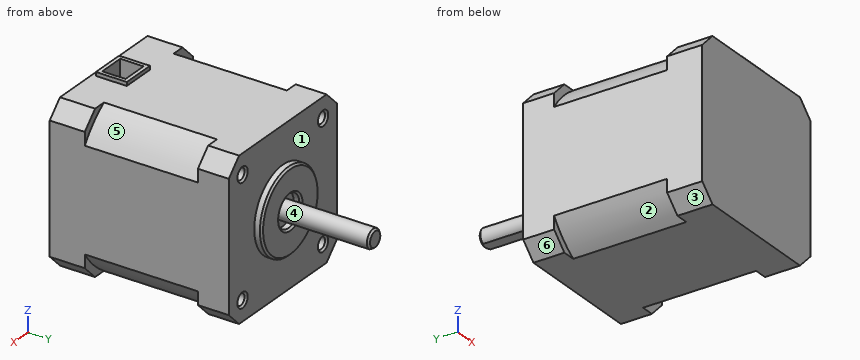
from build123d import *

# Parameters (mm, degrees)
SKETCH1_W           = 42
SKETCH1_H           = 42
BOSS_EXTRUDE1_DEPTH = 47.5
CHAMFER1_SIZE       = 4
SKETCH2_R           = 11.1
SKETCH2_R_2         = 4.25
BOSS_EXTRUDE2_DEPTH = 2
SKETCH4_R           = 2.5
BOSS_EXTRUDE3_DEPTH = 24.5
CHAMFER2_SIZE       = 0.5
CUT_EXTRUDE1_DEPTH  = 18
SKETCH6_R           = 1.5
CUT_EXTRUDE2_DEPTH  = 5
CUT_EXTRUDE3_START  = 9.3
SKETCH7_R           = 36.852304789
SKETCH7_R_2         = 25
CUT_EXTRUDE3_DEPTH  = 30
SKETCH8_W           = 9
SKETCH8_H           = 8.197254607
SKETCH8_W_2         = 7
SKETCH8_H_2         = 6.197254607
EXTRUDE_THIN1_DEPTH = 1
SKETCH9_W           = 7
SKETCH9_H           = 6.197254607
CUT_EXTRUDE4_DEPTH  = 5
CHAMFER3_SIZE       = 0.5


with BuildPart() as part:
    # Sketch1 → Boss-Extrude1 (new body)
    with BuildSketch(Plane(origin=(0, 0, 0), x_dir=(1, 0, 0), z_dir=(0, 1, 0))):
        Rectangle(SKETCH1_W, SKETCH1_H)
    extrude(amount=BOSS_EXTRUDE1_DEPTH)

    # Chamfer1
    chamfer1_edges = [part.edges().sort_by_distance(p)[0] for p in [
        (21, 23.75, 21),
        (-21, 23.75, 21),
        (-21, 23.75, -21),
        (21, 23.75, -21),
    ]]
    chamfer(chamfer1_edges, length=CHAMFER1_SIZE)

    # Sketch2 → Boss-Extrude2 (add)
    with BuildSketch(Plane.XZ.offset(-47.5)):
        with Locations(Location((0, 0, 0), (0, 0, 270))):
            Circle(SKETCH2_R)
        with Locations(Location((0, 0, 0), (0, 0, 270))):
            Circle(SKETCH2_R_2, mode=Mode.SUBTRACT)
    extrude(amount=-BOSS_EXTRUDE2_DEPTH)

    # Sketch4 → Boss-Extrude3 (add)
    with BuildSketch(Plane(origin=(0, 47.5, 0), x_dir=(1, 0, 0), z_dir=(0, 1, 0))):
        with Locations(Location((0, 0, 0), (0, 0, 270))):
            Circle(SKETCH4_R)
    extrude(amount=BOSS_EXTRUDE3_DEPTH)

    # Chamfer2
    chamfer2_edges = [part.edges().sort_by_distance(p)[0] for p in [
        (0, 72, -2.5),
    ]]
    chamfer(chamfer2_edges, length=CHAMFER2_SIZE)

    # Sketch5 → Cut-Extrude1 (cut)
    with BuildSketch(Plane(origin=(0, 72, 0), x_dir=(1, 0, 0), z_dir=(0, 1, 0))):
        Polygon((-1.867188484, 2), (1.973628394, 2), (0.053219955, 2.996371605), align=None)
    extrude(amount=-CUT_EXTRUDE1_DEPTH, mode=Mode.SUBTRACT)

    # Sketch6 → Cut-Extrude2 (cut)
    with BuildSketch(Plane(origin=(0, 47.5, 0), x_dir=(1, 0, 0), z_dir=(0, 1, 0))):
        with Locations(Location((-15.637811111, 15.662146765, 0), (0, 0, 270))):
            Circle(SKETCH6_R)
        with Locations(Location((15.662146765, 15.637811111, 0), (0, 0, 270))):
            Circle(SKETCH6_R)
        with Locations(Location((15.637811111, -15.662146765, 0), (0, 0, 270))):
            Circle(SKETCH6_R)
        with Locations(Location((-15.662146765, -15.637811111, 0), (0, 0, 270))):
            Circle(SKETCH6_R)
    extrude(amount=-CUT_EXTRUDE2_DEPTH, mode=Mode.SUBTRACT)

    # Sketch7 → Cut-Extrude3 (cut)
    with BuildSketch(Plane(origin=(0, 0, 0), x_dir=(1, 0, 0), z_dir=(0, 1, 0)).offset(CUT_EXTRUDE3_START)):
        Circle(SKETCH7_R)
        Circle(SKETCH7_R_2, mode=Mode.SUBTRACT)
    extrude(amount=CUT_EXTRUDE3_DEPTH, mode=Mode.SUBTRACT)

    # Sketch8 → Extrude-Thin1 (add)
    with BuildSketch(Plane.XY.offset(21)):
        with Locations((0, 5.081594665)):
            Rectangle(SKETCH8_W, SKETCH8_H)
        with Locations((0, 5.081594665)):
            Rectangle(SKETCH8_W_2, SKETCH8_H_2, mode=Mode.SUBTRACT)
    extrude(amount=EXTRUDE_THIN1_DEPTH)

    # Sketch9 → Cut-Extrude4 (cut)
    with BuildSketch(Plane.XY.offset(21)):
        with Locations((0, 5.081594665)):
            Rectangle(SKETCH9_W, SKETCH9_H)
    extrude(amount=-CUT_EXTRUDE4_DEPTH, mode=Mode.SUBTRACT)

    # Chamfer3
    chamfer3_edges = [part.edges().sort_by_distance(p)[0] for p in [
        (0, 49.5, 11.1),
        (0, 49.5, 4.25),
        (-15.637811111, 47.5, -17.162146765),
        (15.662146765, 47.5, -17.137811111),
        (15.637811111, 47.5, 14.162146765),
        (-15.662146765, 47.5, 14.137811111),
    ]]
    chamfer(chamfer3_edges, length=CHAMFER3_SIZE)


solid = part.part
Source: CAD feature listing. Evaluate the final solid. Frame: model axes, mm. Face numbers are marked on the shaded views. A direction names the side the tool comes from. Round coordinates to 2 decimals unless told otherwise and drop trailing zeros. Loops run counter-clockwise (first coordinate to the right, second up) from the corner with the lowest first, then second, coordinate; pieces in that order, holes last. Notation, with made-up numbers: (1.5, 28) - (40.5, 28) arc R21 cw to (40.5, 54) - close; hole circle Ø7 at (71, 22.5). An arc over 180 degrees is marked (long way). Write item = value, one per line. Start each with the question number.
(1) Pull-direction query (Y, two-part tool) for the marked faces 1, 2 and 3; classes: +Y half, -Y half, draft (parallel to the pull), parting line (faces both ways), or undercut.
(2) Pin query (flat end, axial travel): pin 1 (12 mm diameter, centred on x = 12, z = -9.5, fed in from +Y); pin 2 (12 mm diameter, centred on y = 57.5, z = -13, fed in from -X); pin 3 (1.1 mm diameter, centred on y = 6.5, z = 21.5, fed in from -X); pin 4 (1.5 mm diameter, centred on x = -15.5, z = 16, fed in from +Y). Return the tip coordinate at first contact, or that it passes through.
(3) Section query A-A, the plane y = 26.5. Output: boundary loops of the cut face in (x, z), plus the area to 3 significant figures.
(4) Section query B-B, the plane z = 0. Output: boundary loops of the cut face in (x, y), plus the area to 3 significant figures.
(5) Ray query, line 1 along X through (y, z) = (48, 0); line 2 along Y through (x, z) = (-14, 1); line 3 along Y through (x, z) = (-7.5, -7). Return the intervals inside material, ascending. Write a range as from..to.
(6) Set-up query: the marked faces 4, 5 and 6. Return all of +Z, -Z, +X, -X, +Y, -Y with unobstructed straight access to the full face (end or side cutting, diameter ignored); none if empty.
Conclusion:
q1.face_1 = +Y half
q1.face_2 = undercut
q1.face_3 = draft
q2.pin_1 = 49.5
q2.pin_2 = through
q2.pin_3 = -17.05
q2.pin_4 = 42.5
q3.outline = (-21, -13.56) arc R25 ccw to (-13.56, -21) - (13.56, -21) arc R25 ccw to (21, -13.56) - (21, 13.56) arc R25 ccw to (13.56, 21) - (-13.56, 21) arc R25 ccw to (-21, 13.56) - close
q3.area = 1,670 mm2
q4.outline = (-21, 0) - (21, 0) - (21, 47.5) - (11.1, 47.5) - (11.1, 49) - (10.6, 49.5) - (4.75, 49.5) - (4.25, 49) - (4.25, 47.5) - (2.5, 47.5) - (2.5, 71.5) - (2, 72) - (-2, 72) - (-2.5, 71.5) - (-2.5, 47.5) - (-4.25, 47.5) - (-4.25, 49) - (-4.75, 49.5) - (-10.6, 49.5) - (-11.1, 49) - (-11.1, 47.5) - (-21, 47.5) - close
q4.area = 2,140 mm2
q5.line_1 = -11.1..-4.25, -2.5..2.5, 4.25..11.1
q5.line_2 = 0..47.5
q5.line_3 = 0..49.5
q6.face_4 = +Y
q6.face_5 = +Z, +X
q6.face_6 = -Z, -X, +Y, -Y
